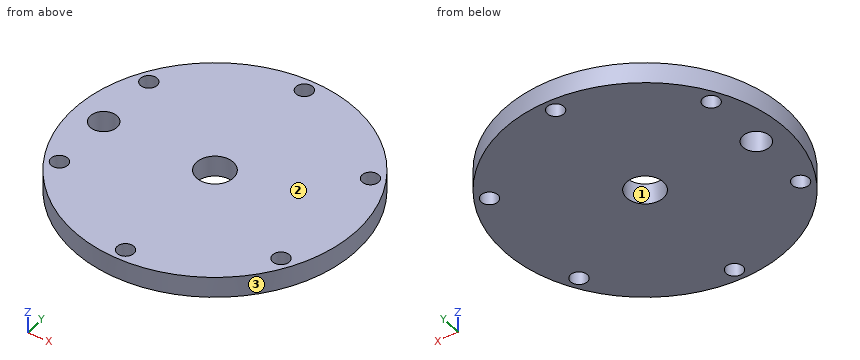
Autodesk Inventor part; units mm, degrees
ref_plane "YZ Plane" through (0, 0, 0) normal (1, 0, 0) x (0, 1, 0)
ref_plane "XZ Plane" through (0, 0, 0) normal (0, 1, 0) x (-1, 0, 0)
ref_plane "XY Plane" through (0, 0, 0) normal (0, 0, 1) x (1, 0, 0)
sketch "Sketch1" plane through (0, 0, 0) normal (0, 0, 1) x (1, 0, 0)
  circle A0 centre (0, 0) radius 32.1945
  dimension "d0" = 64.389
extrude "Extrusion1" add sketch "Sketch1" along normal blind 4.7625
sketch "Sketch2" plane through (0, 0, 4.7625) normal (0, 0, 1) x (1, 0, 0)
  line L0 (0, 0) -> (0, 29.21)
  circle A0 centre (0, 29.21) radius 1.905
  circle A1 centre (-25.2966, 14.605) radius 1.905
  circle A2 centre (-25.2966, -14.605) radius 1.905
  circle A3 centre (0, -29.21) radius 1.905
  circle A4 centre (25.2966, -14.605) radius 1.905
  circle A5 centre (25.2966, 14.605) radius 1.905
  dimension "d3" = 29.21
  dimension "d4" = 3.81
  dimension "d7" = 360
extrude "Extrusion2" cut sketch "Sketch2" against normal through all
sketch "Sketch4" plane through (0, 0, 0) normal (0, 0, -1) x (-1, 0, 0)
  line L0 (0, 0) -> (25.4, 0)
  line L1 (20.0474, 0) -> (22.7237, 4.6355)
  line L2 (22.7237, 4.6355) -> (28.0763, 4.6355)
  line L3 (28.0763, 4.6355) -> (30.7526, 0)
  line L4 (30.7526, 0) -> (28.0763, -4.6355)
  line L5 (28.0763, -4.6355) -> (22.7237, -4.6355)
  line L6 (22.7237, -4.6355) -> (20.0474, 0)
  dimension "d12" = 25.4
  dimension "d13" = 9.271
extrude "Extrusion3" cut sketch "Sketch4" against normal through all
sketch "Sketch5" plane through (0, 0, 0) normal (0, 0, -1) x (-1, 0, 0)
  line L0 (22.7237, -4.6355) -> (20.0474, 0)
  line L1 (20.0474, 0) -> (22.7237, 4.6355)
  line L2 (22.7237, 4.6355) -> (28.0763, 4.6355)
  line L3 (28.0763, 4.6355) -> (30.7526, 0)
  line L4 (30.7526, 0) -> (28.0763, -4.6355)
  line L5 (28.0763, -4.6355) -> (22.7237, -4.6355)
  circle A0 centre (0, 0) radius 32.1945
  circle A1 centre (25.4, 0) radius 3.048
  line L6 (0, 0) -> (25.4, 0)
  dimension "d16" = 6.096
  dimension "d22" = 25.4
extrude "Extrusion4" add sketch "Sketch5" against normal up to surface (4.7625 mm away) contours L0 L1 L2 L3 L4 L5
sketch "Sketch6" plane through (0, 0, 4.7625) normal (0, 0, 1) x (1, 0, 0)
  circle A0 centre (0, 0) radius 4.191
  dimension "d19" = 8.382
extrude "Extrusion5" cut sketch "Sketch6" against normal through all
properties part number "pistonSealingDisc" material "Aluminum 6061"
Verification items for the finished model (mm, model axes). Face numbers are marked on the shaded views. Give positions to 0.01 mm unless a question says otherwise; leave off trailing zeros. Order: outer loops, then holes, each group sorted by start corner. A loop starts at its lowest first (then second) coordinate and runs counter-clockwise, first axis right, second up. Notation, with made-up numbers: (-37.75, 88) -> (-18.75, 88) arc R23 cw to (-18.75, 101) -> close; hole circle Ø10 at (-13.5, -24). An arc over 180 degrees is marked (long way). Use a Markdown table: item, result.
1) Material ranges on probe 1 along Y at (x, z) = (0, 3.6) (1 decimal); probe 2 along X at (y, z) = (13.5, 0.85); probe 3 along X at (y, z) = (13, 1.5), recorded low to high.
Results:
| item | result |
|---|---|
| probe 1 | -32.2 to -31.1, -27.3 to -4.2, 4.2 to 27.3, 31.1 to 32.2 |
| probe 2 | -29.23 to -26.85, -23.74 to 23.74, 26.85 to 29.23 |
| probe 3 | -29.45 to -26.32, -24.27 to 24.27, 26.32 to 29.45 |
2) Section check C-C, the plane z = 2.8. Give the number of separate pieces and of enclosed holes in the cut face, then the cut area to 3 significant figures.
Results:
| item | result |
|---|---|
| separate pieces | 1 |
| enclosed holes | 8 |
| area | 3,100 mm² |
3) Section check D-D, the plane x = -25. Record the boundary of the cut face in (y, z), then the cut area to 3 significant figures.
Results:
| item | result |
|---|---|
| outline | (-20.29, 0) -> (-16.49, 0) -> (-16.49, 4.76) -> (-20.29, 4.76) -> close; (-12.72, 0) -> (-3.02, 0) -> (-3.02, 4.76) -> (-12.72, 4.76) -> close; (3.02, 0) -> (12.72, 0) -> (12.72, 4.76) -> (3.02, 4.76) -> close; (16.49, 0) -> (20.29, 0) -> (20.29, 4.76) -> (16.49, 4.76) -> close |
| area | 129 mm² |
4) Depth check by flat-ended pin: pin 1 Ø3.5 at (x, y) = (0, 29.21) entering from -Z. Enter the tip coordinate at first touch or a pass-through.
Results:
| item | result |
|---|---|
| pin 1 | through |
5) Mould release check, pull along X, two halves, no side actions. Record for the marked faces 1, 2 and 3: pulls with the +X half, pulls with the -X half, needs draft (parallel to the pull), parting line crosses it, or undercut.
Results:
| item | result |
|---|---|
| face 1 | undercut |
| face 2 | needs draft |
| face 3 | parting line crosses it |
6) Section check B-B, the plane y = 29.21. Record the boundary of the cut face in (x, z) (1 decimal).
Results:
| item | result |
|---|---|
| outline | (-13.5, 0) -> (-1.9, 0) -> (-1.9, 4.8) -> (-13.5, 4.8) -> close; (1.9, 0) -> (13.5, 0) -> (13.5, 4.8) -> (1.9, 4.8) -> close |
7) Section check A-A, the plane x = 0. Record the boundary of the cut face in (y, z) (1 decimal), then the cut area to 3 significant figures.
Results:
| item | result |
|---|---|
| outline | (-32.2, 0) -> (-31.1, 0) -> (-31.1, 4.8) -> (-32.2, 4.8) -> close; (-27.3, 0) -> (-4.2, 0) -> (-4.2, 4.8) -> (-27.3, 4.8) -> close; (4.2, 0) -> (27.3, 0) -> (27.3, 4.8) -> (4.2, 4.8) -> close; (31.1, 0) -> (32.2, 0) -> (32.2, 4.8) -> (31.1, 4.8) -> close |
| area | 230 mm² |
